```python
from build123d import *

# Parameters (mm, degrees)
F0_R     = 7.14375
F1_DEPTH = 6.35


with BuildPart() as f1:
    # F0 (on Front) → F1 (new body)
    with BuildSketch(Plane.XZ):
        with BuildLine():
            ThreePointArc((-171.45, 127), (-175.940128, 125.140128), (-177.8, 120.65))
            Line((-177.8, 120.65), (-177.8, -20.6375))
            Line((-177.8, -20.6375), (-177.8, -30.1625))
            Line((-177.8, -30.1625), (-177.8, -120.65))
            ThreePointArc((-177.8, -120.65), (-175.940128, -125.140128), (-171.45, -127))
            Line((-171.45, -127), (171.45, -127))
            ThreePointArc((171.45, -127), (175.940128, -125.140128), (177.8, -120.65))
            Line((177.8, -120.65), (177.8, -30.1625))
            Line((177.8, -30.1625), (177.8, -20.6375))
            Line((177.8, -20.6375), (177.8, 120.65))
            ThreePointArc((177.8, 120.65), (175.940128, 125.140128), (171.45, 127))
            Line((171.45, 127), (-171.45, 127))
        make_face()
        with Locations((-139.746101, -88.850368)):
            Circle(F0_R, mode=Mode.SUBTRACT)
        with Locations((139.713767, -88.917399)):
            Circle(F0_R, mode=Mode.SUBTRACT)
        with Locations((-50.802743, 4.775175)):
            Circle(F0_R, mode=Mode.SUBTRACT)
        with Locations((-139.7, 88.9)):
            Circle(F0_R, mode=Mode.SUBTRACT)
        with Locations((50.814427, 4.760493)):
            Circle(F0_R, mode=Mode.SUBTRACT)
        with Locations((139.654712, 88.858014)):
            Circle(F0_R, mode=Mode.SUBTRACT)
    extrude(amount=F1_DEPTH)


solid = f1.part
```
Part model, mm, in its own coordinate system. Round coordinates to 2 decimals unless told otherwise and drop trailing zeros. Loops run counter-clockwise (first coordinate to the right, second up) from the corner with the lowest first, then second, coordinate; pieces in that order, holes last.
1. Drill centre lines: line 1 along Z through (x, y) = (-143, -3.75); line 2 along X through (y, z) = (-3.25, 7.5). Where is each one in solid material? Low to high.
Solutions:
line 1: z = -127 to -95.21, -82.49 to 82.56, 95.24 to 127
line 2: x = -177.8 to -57.41, -44.2 to 44.22, 57.41 to 177.8
2. Two-plate mould, pull along Z, no slides. Class faces 1 (the face through (-2, -6.35, 2)), 2 (the face through (-57.94, -3.13, 5.09)): pulls with the +Z half, pulls with the -Z half, needs draft (parallel to the pull), parting line crosses it, or undercut.
Solutions:
face 1: needs draft
face 2: undercut
3. Slice it at A-A (x = -139.7). Give the cut face in (y, z), and give its area (3 significant figures).
Solutions:
outline: (-6.35, -127) - (0, -127) - (0, -95.99) - (-6.35, -95.99) - close; (-6.35, -81.71) - (0, -81.71) - (0, 81.76) - (-6.35, 81.76) - close; (-6.35, 96.04) - (0, 96.04) - (0, 127) - (-6.35, 127) - close
area: 1,430 mm2
